Work out the finished part from the listing and answer in its coordinate system (mm). Face numbers are marked on the shaded views. A direction names the side the tool comes from. Coordinates: 2 decimals unless noted, no trailing zeros. Order: outer loops, then holes, each group sorted by start corner. A loop starts at its lowest first (then second) coordinate and runs counter-clockwise, first axis right, second up. Notation, with made-up numbers: (36.5, 14.25) -> (87.5, 14.25) arc R19 cw to (87.5, 30.25) -> close; hole circle Ø1 at (67.5, -28). An arc over 180 degrees is marked (long way). Answer as CSV lines item,"result". Start each with the question number.
Item 1: Section D-D (y = 0) is taken. Write down the section's boundary in (x, z).
Item 2: For a pull along X with two mould halves and no side action, classify the marked faces 1, 2, 3 and 4 as pulls with the +X half, pulls with the -X half, needs draft (parallel to the pull), parting line crosses it, or undercut.
Item 3: Each of these flat-tipped pins is pushed along its axis until it touches: pin 1 Ø4 at (x, y) = (-16, 0.5) entering from +Z; pin 2 Ø8 at (y, z) = (24.5, 11.5) entering from -X; pin 3 Ø5.5 at (x, z) = (-31, 13) entering from +Y; pin 4 Ø7.5 at (x, z) = (30, 10) entering from +Y. Where does it stop, or does it pass through?
Item 4: Which of the six approach directions +Z, -Z, +X, -X, +Y, -Y give full straight-line access (tool end or side, diameter ignored) to the marked faces 5, 6 and 7?
Item 5: Straight lines are drawn through the part: L1, parallel to Y at x = 24.5, z = 12.75; L2, parallel to Y at x = 15.5, z = 12.5; L3, parallel to Z at x = -32, y = 0. For each, find the intervals that lie inside material, in ascending order.
Item 6: Section A-A (x = 0) is taken. Write down the section's boundary in (y, z).
Item 7: Section B-B (y = -25) is taken. Write down the section's boundary in (x, z), then the cut area to 3 significant figures.
Item 8: Section C-C (z = 12.5) is taken. Write down the section's boundary in (x, y), then the cut area to 3 significant figures.
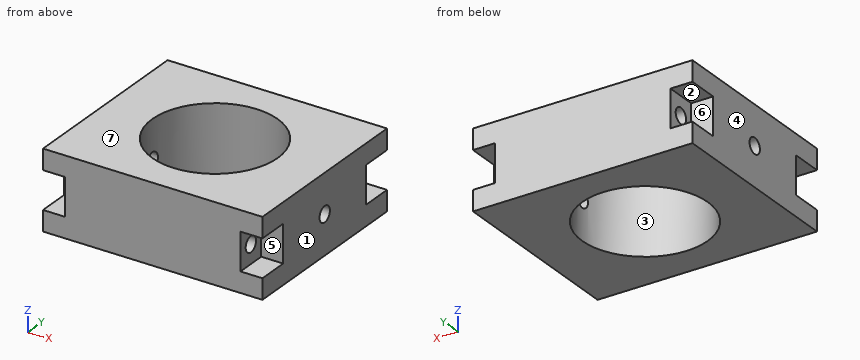
```python
from build123d import *

# Parameters (mm, degrees)
SKETCH1_W           = 70
SKETCH1_H           = 60
SKETCH1_R           = 20
BOSS_EXTRUDE1_DEPTH = 25
SKETCH2_R           = 2.5
CUT_EXTRUDE1_DEPTH  = 81.156097709
SKETCH3_W           = 7
SKETCH3_H           = 12
CUT_EXTRUDE2_DEPTH  = 10


with BuildPart() as part:
    # Sketch1 → Boss-Extrude1 (new body)
    with BuildSketch(Plane.XY):
        Rectangle(SKETCH1_W, SKETCH1_H)
        Circle(SKETCH1_R, mode=Mode.SUBTRACT)
    extrude(amount=BOSS_EXTRUDE1_DEPTH)

    # Sketch2 → Cut-Extrude1 (cut, through all)
    with BuildSketch(Plane(origin=(35, 0, 0), x_dir=(0, 0, -1), z_dir=(1, 0, 0))):
        with Locations((-12.5, 25)):
            Circle(SKETCH2_R)
        with Locations((-12.5, -25)):
            Circle(SKETCH2_R)
        with Locations((-12.5, 0)):
            Circle(SKETCH2_R)
    extrude(amount=-CUT_EXTRUDE1_DEPTH, mode=Mode.SUBTRACT)

    # Sketch3 → Cut-Extrude2 (cut)
    with BuildSketch(Plane(origin=(0, 30, 0), x_dir=(1, 0, 0), z_dir=(0, 1, 0))):
        Polygon((-28, -6.5), (-35, -6.5), (-35, -18.5), (-28, -18.5), (-28, -15), (-28, -10), align=None)
        with Locations((31.5, -12.5)):
            Rectangle(SKETCH3_W, SKETCH3_H)
    cut_extrude2 = extrude(amount=-CUT_EXTRUDE2_DEPTH, mode=Mode.SUBTRACT)

    # Mirror1: Cut-Extrude2 across plane
    add(cut_extrude2.mirror(Plane.ZX), mode=Mode.SUBTRACT)


solid = part.part
```
Checked values:
1,outline,"(-35, 0) -> (-20, 0) -> (-20, 10) -> (-35, 10) -> close; (-35, 15) -> (-20, 15) -> (-20, 25) -> (-35, 25) -> close; (20, 0) -> (35, 0) -> (35, 10) -> (20, 10) -> close; (20, 15) -> (35, 15) -> (35, 25) -> (20, 25) -> close"
2,face 1,"pulls with the +X half"
2,face 2,"needs draft"
2,face 3,"undercut"
2,face 4,"pulls with the -X half"
3,pin 1,"passes through"
3,pin 2,"stops at x = -28"
3,pin 3,"stops at y = 20"
3,pin 4,"stops at y = 30"
4,face 5,"+X, -Y"
4,face 6,"-X, +Y"
4,face 7,"+Z, +X, -X, +Y, -Y"
5,L1,"y = -30 to -27.49, -22.51 to -2.49, 2.49 to 22.51, 27.49 to 30"
5,L2,"y = -30 to -27.5, -22.5 to -12.64, 12.64 to 22.5, 27.5 to 30"
5,L3,"z = 0 to 10, 15 to 25"
6,outline,"(-30, 0) -> (-20, 0) -> (-20, 25) -> (-30, 25) -> close; (20, 0) -> (30, 0) -> (30, 25) -> (20, 25) -> close; hole circle Ø5 at (-25, 12.5); hole circle Ø5 at (25, 12.5)"
7,outline,"(-35, 0) -> (35, 0) -> (35, 6.5) -> (28, 6.5) -> (28, 10) -> (-28, 10) -> (-28, 6.5) -> (-35, 6.5) -> close; (-35, 18.5) -> (-28, 18.5) -> (-28, 15) -> (28, 15) -> (28, 18.5) -> (35, 18.5) -> (35, 25) -> (-35, 25) -> close"
7,area,"1,300 mm^2"
8,outline,"(-35, -20) -> (-28, -20) -> (-28, -22.5) -> (28, -22.5) -> (28, -20) -> (35, -20) -> (35, -2.5) -> (19.84, -2.5) arc R20 cw to (-19.84, -2.5) -> (-35, -2.5) -> close; (-35, 2.5) -> (-19.84, 2.5) arc R20 cw to (19.84, 2.5) -> (35, 2.5) -> (35, 20) -> (28, 20) -> (28, 22.5) -> (-28, 22.5) -> (-28, 20) -> (-35, 20) -> close; (-28, -30) -> (28, -30) -> (28, -27.5) -> (-28, -27.5) -> close; (-28, 27.5) -> (28, 27.5) -> (28, 30) -> (-28, 30) -> close"
8,area,"1,950 mm^2"
